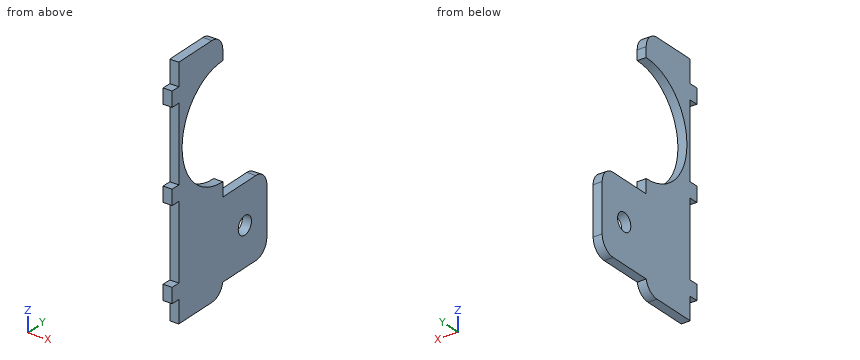
```python
from build123d import *

# Parameters (mm, degrees)
SKETCH1_W           = 80
SKETCH1_H           = 40
BOSS_EXTRUDE1_DEPTH = 3
SKETCH8_R           = 3
SKETCH8_W           = 4
SKETCH8_H           = 20
CUT_EXTRUDE4_DEPTH  = 54.761045377
FILLET1_R           = 5
SKETCH3_W           = 3
SKETCH3_H           = 5
BOSS_EXTRUDE2_DEPTH = 3
LPATTERN1_COUNT     = 3
LPATTERN1_PITCH     = 30


with BuildPart() as part:
    # Sketch1 → Boss-Extrude1 (new body)
    with BuildSketch(Plane(origin=(0, 0, 0), x_dir=(0, 0, -1), z_dir=(1, 0, 0))):
        with Locations((-7.5, -5)):
            Rectangle(SKETCH1_W, SKETCH1_H)
    extrude(amount=BOSS_EXTRUDE1_DEPTH)

    # Sketch8 → Cut-Extrude4 (cut, through all)
    with BuildSketch(Plane.ZY):
        with Locations((-15.5, 5)):
            Circle(SKETCH8_R)
        with BuildLine():
            Line((39.2, -5), (47.5, -5))
            Line((47.5, -5), (47.5, 15))
            Line((47.5, 15), (39.2, 15))
            Line((39.2, 15), (2.2, 15))
            Line((2.2, 15), (-2.5, 15))
            Line((-2.5, 15), (-2.5, -5))
            Line((-2.5, -5), (2.2, -5))
            ThreePointArc((2.2, -5), (20.7, -23.5), (39.2, -5))
        make_face()
        with Locations((-30.5, 5)):
            Rectangle(SKETCH8_W, SKETCH8_H)
    extrude(amount=-CUT_EXTRUDE4_DEPTH, mode=Mode.SUBTRACT)

    # Fillet1
    # the kernel refuses this fillet: 5 mm, written as the material it takes off along each edge
    with BuildSketch(Plane(origin=(-12.5, -5, 47.5), x_dir=(0, -1, 0), z_dir=(1, 0, 0)), Plane(origin=(-12.5, 15, -28.5), x_dir=(0, 0, 1), z_dir=(1, 0, 0))) as fillet1_piece_1:
        with BuildLine():
            CenterArc((FILLET1_R, FILLET1_R), FILLET1_R, 180, 90)
            Line((0, FILLET1_R), (-FILLET1_R * 0.02, FILLET1_R))
            Line((-FILLET1_R * 0.02, FILLET1_R), (-FILLET1_R * 0.02, -FILLET1_R * 0.02))
            Line((-FILLET1_R * 0.02, -FILLET1_R * 0.02), (FILLET1_R, -FILLET1_R * 0.02))
            Line((FILLET1_R, -FILLET1_R * 0.02), (FILLET1_R, 0))
        make_face()
    extrude(amount=28, mode=Mode.SUBTRACT)
    with BuildSketch(Plane(origin=(-12.5, 15, -2.5), x_dir=(0, 0, -1), z_dir=(1, 0, 0))) as fillet1_piece_2:
        with BuildLine():
            CenterArc((FILLET1_R, -FILLET1_R), FILLET1_R, 90, 90)
            Line((0, -FILLET1_R), (-FILLET1_R * 0.02, -FILLET1_R))
            Line((-FILLET1_R * 0.02, -FILLET1_R), (-FILLET1_R * 0.02, FILLET1_R * 0.02))
            Line((-FILLET1_R * 0.02, FILLET1_R * 0.02), (FILLET1_R, FILLET1_R * 0.02))
            Line((FILLET1_R, FILLET1_R * 0.02), (FILLET1_R, 0))
        make_face()
    extrude(amount=28, mode=Mode.SUBTRACT)
    with BuildSketch(Plane(origin=(-12.247448714, -5, -32.5), x_dir=(0, -1.5645262863012704e-12, 1.0), z_dir=(1, 0, 0))) as fillet1_piece_3:
        with BuildLine():
            CenterArc((5, 4.898979486), FILLET1_R, 180, 78.463040967)
            Line((0, 4.898979486), (-0.1, 4.898979486))
            Line((-0.1, 4.898979486), (-0.1, 0))
            Line((-0.1, 0), (0, -0.1))
            ThreePointArc((0, -0.1), (2, -0.1), (3.98, -0.09797959))
            Line((3.98, -0.09797959), (4, 0))
        make_face()
    extrude(amount=27.494897428, mode=Mode.SUBTRACT)

    # Sketch3 → Boss-Extrude2 (add)
    with BuildSketch(Plane.XZ.offset(25)):
        with Locations((1.5, 37.5)):
            Rectangle(SKETCH3_W, SKETCH3_H)
    boss_extrude2 = extrude(amount=BOSS_EXTRUDE2_DEPTH)

    # LPattern1: Boss-Extrude2 ×3
    with Locations(*[(0, 0, -i * LPATTERN1_PITCH) for i in range(1, LPATTERN1_COUNT)]):
        add(boss_extrude2)


solid = part.part
```
The model under review builds one solid part; all positions refer to its coordinate system, in mm. Coordinates: 2 decimals unless noted, no trailing zeros. Write each loop counter-clockwise with the first axis right and the second up, starting at its lowest first coordinate (ties: lowest second). Pieces come first, ordered by that corner, then holes.
1) To check wall thickness, follow probe 1 along Y at (x, z) = (1.1, -15.5); probe 2 along Z at (x, y) = (2.6, 5.5); probe 3 along Z at (x, y) = (2, 1.5). State the ranges of each line that lie inside material, in increasing order.
2) We need section B-B on y = -15. State the section outline as (x, z) points.
3) We need section C-C on x = 1.6. State the section outline as (y, z) points, then the cut area to 3 significant figures.
4) We need section D-D on y = -0.5. State the section outline as (x, z) points, then the cut area to 3 significant figures.
5) We need section A-A on z = -15.5. State the section outline as (x, y) points, then the cut area to 3 significant figures.
6) Clearance check with flat-ended pins moving along their axes: pin 1 Ø0.9 at (x, z) = (1.5, 23) entering from -Y; pin 2 Ø0.9 at (x, y) = (1, -26.5) entering from -Z; pin 3 Ø0.9 at (x, y) = (1.5, 3.5) entering from +Z; pin 4 Ø3.5 at (y, z) = (5, -15.5) entering from +X. State where each tip first meets the part, or that it passes through.
Answer list:
1. probe 1: y = -25 to 2, 8 to 15
1. probe 2: z = -28.5 to -18.46, -12.54 to -2.5
1. probe 3: z = -28.5 to -2.5
2. outline: (0, -32.5) - (3, -32.5) - (3, 5.14) - (0, 5.14) - close; (0, 36.26) - (3, 36.26) - (3, 47.5) - (0, 47.5) - close
3. outline: (-28, -25) - (-25, -25) - (-25, -32.5) - (-9.9, -32.5) arc R5 ccw to (-5, -28.5) - (10, -28.5) arc R5 ccw to (15, -23.5) - (15, -7.5) arc R5 ccw to (10, -2.5) - (-5, -2.5) - (-5, 2.2) arc R18.5 cw to (-5, 39.2) - (-5, 42.5) arc R5 ccw to (-10, 47.5) - (-25, 47.5) - (-25, 40) - (-28, 40) - (-28, 35) - (-25, 35) - (-25, 10) - (-28, 10) - (-28, 5) - (-25, 5) - (-25, -20) - (-28, -20) - close; hole circle Ø6 at (5, -15.5)
3. area: 1,580 mm2
4. outline: (0, -28.5) - (3, -28.5) - (3, -2.5) - (0, -2.5) - close
4. area: 78.0 mm2
5. outline: (0, -25) - (3, -25) - (3, 2) - (0, 2) - close; (0, 8) - (3, 8) - (3, 15) - (0, 15) - close
5. area: 102 mm2
6. pin 1: stops at y = -25
6. pin 2: stops at z = -25
6. pin 3: stops at z = -2.5
6. pin 4: passes through
